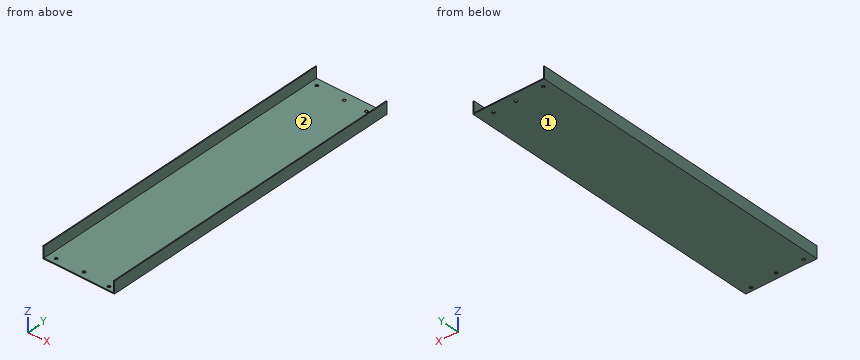
```python
from build123d import *

# Parameters (mm, degrees)
F1_DEPTH = 660
F3_D     = 6.35


with BuildPart() as f1:
    # F0 (on Front) → F1 (new body)
    with BuildSketch(Plane.XZ):
        Polygon((0, -23), (0, 0), (-2, 0), (-2, -25), (148, -25), (148, 0), (146, 0), (146, -23), align=None)
    extrude(amount=F1_DEPTH)

    # F3 (through all)
    with Locations(Plane.XY.offset(-23)):
        with Locations((15.7224, -648.32902), (73, -647.237599), (129.395574, -651.889563), (120.003812, -17.314114), (73, -17.314114), (13.673902, -15.054441)):
            Hole(F3_D / 2)


solid = f1.part
```
Could you check a few things on this model? Use its own coordinates, in mm. Face numbers are marked on the shaded views. Coordinates: 2 decimals unless noted, no trailing zeros. Write each loop counter-clockwise with the first axis right and the second up, starting at its lowest first coordinate (ties: lowest second). Pieces come first, ordered by that corner, then holes. Notation, with made-up numbers: (-18.5, 25) -> (38.5, 25) arc R21 ccw to (38.5, 63) -> close; hole circle Ø8 at (6.5, 61). An arc over 180 degrees is marked (long way). One line per question, with ' | ' between items. Start each with the question number.
1. If we section it at C-C (x = 90.5): Please give me the cut outline in (y, z).
2. If we section it at B-B (y = -164): Please give me the cut outline in (x, z).
3. Please list where these lines run through material, in increasing order: line 1 along X through (y, z) = (-28, -17.5); line 2 along Z through (x, y) = (14, -160).
4. Will this pin go through, and if not, where does the flat tip stop? P1, Ø7.5, axis at x = 13.67, y = -15.05, coming from the +Z side.
5. Thinking about a two-plate mould opening in X: for the marked faces 1 and 2, which applies, pulls with the +X half, pulls with the -X half, needs draft (parallel to the pull), parting line crosses it, or undercut?
6. If we section it at A-A (z = -7): Please give me the cut outline in (x, y), and give its area (3 significant figures).
Return value:
1) outline: (-660, -25) -> (0, -25) -> (0, -23) -> (-660, -23) -> close
2) outline: (-2, -25) -> (148, -25) -> (148, 0) -> (146, 0) -> (146, -23) -> (0, -23) -> (0, 0) -> (-2, 0) -> close
3) line 1: x = -2 to 0, 146 to 148 | line 2: z = -25 to -23
4) P1: stops at z = -23
5) face 1: needs draft | face 2: undercut
6) outline: (-2, -660) -> (0, -660) -> (0, 0) -> (-2, 0) -> close; (146, -660) -> (148, -660) -> (148, 0) -> (146, 0) -> close | area: 2,640 mm²
